Geometry: final body of the model. Coordinates: model frame, mm. A direction names the side the tool comes from. Give positions to 0.01 mm unless a question says otherwise; leave off trailing zeros. Order: outer loops, then holes, each group sorted by start corner. A loop starts at its lowest first (then second) coordinate and runs counter-clockwise, first axis right, second up. Notation, with made-up numbers: (-17.5, -13.75) - (32.5, -13.75) arc R24 cw to (32.5, 19.25) - close; hole circle Ø9 at (70.25, 51.25). An arc over 180 degrees is marked (long way). Put each result on its own line as item: value. Start each with the question number.
1. Section C-C on y = -40.5. Return the cut outline in (x, z).
2. Set-up query: faces 1 (the flat face through (92.2, -89.8, 15)), 2 (the flat face through (-1, 65, 0)), 3 (the flat face through (-42, -39, -24)), 4 (the flat face through (27.731, 156, -41)). Return all of +Z, -Z, +X, -X, +Y, -Y with unobstructed straight access to the full face (end or side cutting, diameter ignored); none if empty.
3. Ray query, line 1 along Y through (x, z) = (0, 1); line 2 along Y through (x, z) = (0, -35); line 3 along Z through (x, y) = (45, 145). Return the intervals inside material, ascending. Write a range as from..to.
4. Mould query, pull axis X, two halves, no side actions, for faces 5 (the flat face through (-1.25, 153, -63)), 6 (the flat face through (-1, -41, -40)), 7 (the cylindrical face through (-0.544, 174.494, 17.255)). Classes: pulls with the +X half, pulls with the -X half, needs draft (parallel to the pull), parting line crosses it, or undercut.
5. Section B-B on z = -14. Return the cut outline in (x, y).
6. Section D-D on x = -87.5. Return the cut outline in (y, z).
7. First-contact query: P1, Ø1.5, axis at x = -19.5, z = 5.5, coming from the +Y side; P2, Ø12, axis at y = -64.5, z = -14, coming from the -X side; P3, Ø1.5, axis at y = 117, z = -51, coming from the +X side. Flat tips, straight axial feed; report the tip coordinate or a pass-through.
8. Section A-A on x = -6.5. Return the cut outline in (y, z).
from build123d import *

# Parameters (mm, degrees)
F0_R      = 4.5
F1_DEPTH  = 35
F2_DEPTH  = 24
F3_DEPTH  = 15
F5_DEPTH  = 35
F7_DEPTH  = 83
F9_DEPTH  = 290
F10_R     = 18
F11_DEPTH = 199
F12_W     = 2.5
F12_H     = 32
F13_DEPTH = 40
F8_R      = 3.5
F14_DEPTH = 99.1
F15_W     = 76
F15_H     = 160
F16_DEPTH = 16
F17_DEPTH = 24


# Not quite as in the source:
# - a feature names something its author has since deleted; it is built from what else it names


with BuildPart() as f1:
    # F0 (on Top) → F1 (new body)
    with BuildSketch(Plane.XY):
        with BuildLine():
            Line((95, 100), (35, 160))
            Line((35, 160), (-35, 160))
            Line((-35, 160), (-95, 100))
            Line((-95, 100), (-95, -74))
            ThreePointArc((-95, -74), (-83.686291501, -78.686291501), (-79, -90))
            Line((-79, -90), (-79, 40))
            Line((-79, 40), (79, 40))
            Line((79, 40), (79, -90))
            ThreePointArc((79, -90), (83.686291501, -78.686291501), (95, -74))
            Line((95, -74), (95, 100))
        make_face()
        with BuildLine():
            Line((95, -140), (95, -106))
            ThreePointArc((95, -106), (83.686291501, -101.313708499), (79, -90))
            Line((79, -90), (79, -120))
            Line((79, -120), (-79, -120))
            Line((-79, -120), (-79, -90))
            ThreePointArc((-79, -90), (-83.686291501, -101.313708499), (-95, -106))
            Line((-95, -106), (-95, -140))
            Line((-95, -140), (95, -140))
        make_face()
        with BuildLine():
            ThreePointArc((-79, -90), (-83.686291501, -78.686291501), (-95, -74))
            Line((-95, -74), (-95, -106))
            ThreePointArc((-95, -106), (-83.686291501, -101.313708499), (-79, -90))
        make_face()
        with Locations((-87.5, -90)):
            Circle(F0_R, mode=Mode.SUBTRACT)
        with BuildLine():
            Line((95, -106), (95, -74))
            ThreePointArc((95, -74), (83.686291501, -78.686291501), (79, -90))
            ThreePointArc((79, -90), (83.686291501, -101.313708499), (95, -106))
        make_face()
        with Locations((87.5, -90)):
            Circle(F0_R, mode=Mode.SUBTRACT)
        Polygon((79, -120), (79, -90), (79, 40), (-79, 40), (-79, -90), (-79, -120), align=None)
    extrude(amount=F1_DEPTH)

    # F0 (on Top) → F2 (join)
    with BuildSketch(Plane.XY):
        Polygon((79, -120), (79, -90), (79, 40), (-79, 40), (-79, -90), (-79, -120), align=None)
    extrude(amount=-F2_DEPTH)

    # F0 (on Top) → F3 (cut)
    with BuildSketch(Plane.XY):
        with BuildLine():
            ThreePointArc((-79, -90), (-83.686291501, -78.686291501), (-95, -74))
            Line((-95, -74), (-95, -106))
            ThreePointArc((-95, -106), (-83.686291501, -101.313708499), (-79, -90))
        make_face()
        with Locations((-87.5, -90)):
            Circle(F0_R, mode=Mode.SUBTRACT)
        with BuildLine():
            Line((95, -106), (95, -74))
            ThreePointArc((95, -74), (83.686291501, -78.686291501), (79, -90))
            ThreePointArc((79, -90), (83.686291501, -101.313708499), (95, -106))
        make_face()
        with Locations((87.5, -90)):
            Circle(F0_R, mode=Mode.SUBTRACT)
    extrude(amount=F3_DEPTH, mode=Mode.SUBTRACT)

    # F4 (on face) → F5 (join)
    with BuildSketch(Plane(origin=(0, 0, 0), x_dir=(1, 0, 0), z_dir=(0, 0, -1))):
        with BuildLine():
            Line((35, -160), (-35, -160))
            ThreePointArc((-35, -160), (0, -174.4974746831), (35, -160))
        make_face()
    extrude(amount=-F5_DEPTH)

    # F6 (on face) → F7 (join)
    with BuildSketch(Plane(origin=(0, 0, 0), x_dir=(1, 0, 0), z_dir=(0, 0, -1))):
        with BuildLine():
            Line((-27.7308492477, -166), (27.7308492477, -166))
            Line((27.7308492477, -166), (27.7308492477, -150))
            ThreePointArc((27.7308492477, -150), (0, -96.3276844271), (-27.7308492477, -150))
            Line((-27.7308492477, -150), (-27.7308492477, -166))
        make_face()
    extrude(amount=F7_DEPTH)

    # F8 (on face) → F9 (cut)
    with BuildSketch(Plane(origin=(-27.7308492477, 0, 0), x_dir=(0, -1, 0), z_dir=(-1, 0, 0))):
        Polygon((-158, -83), (-166, 0), (-166, -83), align=None)
    extrude(amount=-F9_DEPTH, mode=Mode.SUBTRACT)

    # F10 (on face) → F11 (cut)
    with BuildSketch(Plane(origin=(0, 0, -83), x_dir=(1, 0, 0), z_dir=(0, 0, -1))):
        with Locations((0, -130.3276844271)):
            Circle(F10_R)
    extrude(amount=-F11_DEPTH, mode=Mode.SUBTRACT)

    # F12 (on face) → F13 (cut)
    with BuildSketch(Plane(origin=(0, 0, -83), x_dir=(1, 0, 0), z_dir=(0, 0, -1))):
        with Locations((0, -174)):
            Rectangle(F12_W, F12_H)
        with BuildLine():
            ThreePointArc((1.25, -148.2842291949), (0, -148.3276844271), (-1.25, -148.2842291949))
            Line((-1.25, -148.2842291949), (-1.25, -158))
            Line((-1.25, -158), (1.25, -158))
            Line((1.25, -158), (1.25, -148.2842291949))
        make_face()
    extrude(amount=-F13_DEPTH, mode=Mode.SUBTRACT)

    # F8 (on face) → F14 (cut)
    with BuildSketch(Plane(origin=(-27.7308492477, 0, 0), x_dir=(0, -1, 0), z_dir=(-1, 0, 0))):
        with Locations((-155, -55)):
            Circle(F8_R)
    extrude(amount=-F14_DEPTH, mode=Mode.SUBTRACT)

    # F15 (on face) → F16 (join)
    with BuildSketch(Plane(origin=(0, 0, -24), x_dir=(1, 0, 0), z_dir=(0, 0, -1))):
        Polygon((-46, -40), (-46, 120), (-61, 120), (-79, 102.6506484271), (-79, -22.6506484271), (-61, -40), align=None)
        with Locations((0, 40)):
            Rectangle(F15_W, F15_H)
        Polygon((61, 120), (46, 120), (46, -40), (61, -40), (79, -22.6506484271), (79, 102.6506484271), align=None)
    extrude(amount=F16_DEPTH)

    # F15 (on face) → F17 (cut)
    with BuildSketch(Plane(origin=(0, 0, -24), x_dir=(1, 0, 0), z_dir=(0, 0, -1))):
        Polygon((-79, -40), (-61, -40), (-79, -22.6506484271), align=None)
        Polygon((-79, 102.6506484271), (-61, 120), (-79, 120), align=None)
        Polygon((79, 120), (61, 120), (79, 102.6506484271), align=None)
        Polygon((79, -22.6506484271), (61, -40), (79, -40), align=None)
    extrude(amount=-F17_DEPTH, mode=Mode.SUBTRACT)


solid = f1.part
Resolved:
1. outline: (-95, 0) - (-79, 0) - (-79, -40) - (-46, -40) - (-46, -24) - (-38, -24) - (-38, -40) - (38, -40) - (38, -24) - (46, -24) - (46, -40) - (79, -40) - (79, 0) - (95, 0) - (95, 35) - (-95, 35) - close
2. face 1: -Z, +X
2. face 2: -Z
2. face 3: -Z, +Y, -Y
2. face 4: -Z, +X, +Y
3. line 1: -140..112.33, 148.33..174.5
3. line 2: -120..40, 96.33..112.33, 148.33..162.63
3. line 3: 0..35
4. face 5: undercut
4. face 6: needs draft
4. face 7: parting line crosses it
5. outline: (-79, -102.65) - (-61, -120) - (61, -120) - (79, -102.65) - (79, 22.65) - (61, 40) - (-61, 40) - (-79, 22.65) - close; (-27.73, 150) arc R34 ccw (long way) to (27.73, 150) - (27.73, 164.65) - (-27.73, 164.65) - close; hole circle Ø36 at (0, 130.33)
6. outline: (-140, 0) - (-104.13, 0) - (-104.13, 15) - (-94.5, 15) - (-94.5, 35) - (-140, 35) - close; (-85.5, 15) - (-75.87, 15) - (-75.87, 0) - (107.5, 0) - (107.5, 35) - (-85.5, 35) - close
7. P1: y = 170.81
7. P2: x = -79
7. P3: x = 31.59
8. outline: (-140, 0) - (-120, 0) - (-120, -40) - (40, -40) - (40, 0) - (96.95, 0) - (96.95, -83) - (113.54, -83) - (113.54, 35) - (-140, 35) - close; (147.11, -83) - (158, -83) - (166, 0) - (174.07, 0) - (174.07, 35) - (147.11, 35) - close; hole circle Ø7 at (155, -55)
